Check sheet for the modelled part. Datum: model origin and axes. Units: mm. Coordinates: 2 decimals unless noted, no trailing zeros. Loops run counter-clockwise (first coordinate to the right, second up) from the corner with the lowest first, then second, coordinate; pieces in that order, holes last. Notation, with made-up numbers: M 44,71.5 L 85,71.5 A16 ccw 85,93.5 Z; hole C -32.5,67 d9. An arc over 180 degrees is marked long. Answer in a Markdown table with one row per item. Add a question column.
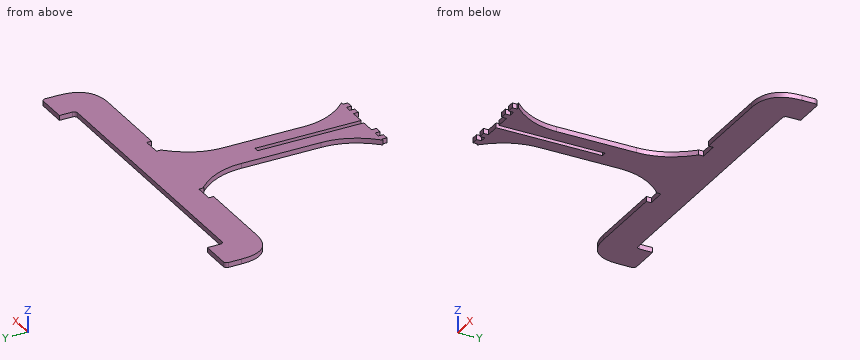
```python
from build123d import *

# Parameters (mm, degrees)
P_IDAT_VYSUNUT_M2_DEPTH  = 3
SKICA2_W                 = 3
SKICA2_H                 = 65
ODEBRAT_VYSUNUT_M3_DEPTH = 3
SKICA3_W                 = 11
SKICA3_H                 = 5.694256757
ODEBRAT_VYSUNUT_M4_DEPTH = 3


with BuildPart() as part:
    # Skica1 → Přidat vysunutím2 (new body)
    with BuildSketch(Plane.XY):
        with BuildLine():
            Line((-90.642636358, 2.694256757), (-30.642636358, 2.694256757))
            add(Edge.make_bspline(
                [(-30.642636358, 2.694256757), (-17.025139471, -11.118063286), (-17.142636358, -27.878389443)],
                knots=[0, 0, 0, 1, 1, 1], degree=2))
            Line((-17.142636358, -27.878389443), (-17.142636358, -76.655981804))
            add(Edge.make_bspline(
                [(-30.642636358, -107.305743243), (-17.009316786, -93.458261678), (-17.142636358, -76.655981804)],
                knots=[0, 0, 0, 1, 1, 1], degree=2))
            Line((-30.642636358, -107.305743243), (-29.497972973, -107.305743243))
            Line((-29.497972973, -107.305743243), (-29.497972973, -110.305743243))
            Line((-29.497972973, -110.305743243), (-25.347972973, -110.305743243))
            Line((-25.347972973, -110.305743243), (-25.347972973, -107.305743243))
            Line((-25.347972973, -107.305743243), (-21.697972973, -107.305743243))
            Line((-21.697972973, -107.305743243), (-21.697972973, -110.305743243))
            Line((-21.697972973, -110.305743243), (-17.547972973, -110.305743243))
            Line((-17.547972973, -110.305743243), (-17.547972973, -107.305743243))
            Line((-17.547972973, -107.305743243), (2.852027027, -107.305743243))
            Line((2.852027027, -107.305743243), (2.852027027, -110.305743243))
            Line((2.852027027, -110.305743243), (7.002027027, -110.305743243))
            Line((7.002027027, -110.305743243), (7.002027027, -107.305743243))
            Line((7.002027027, -107.305743243), (10.652027027, -107.305743243))
            Line((10.652027027, -107.305743243), (10.652027027, -110.305743243))
            Line((10.652027027, -110.305743243), (14.802027027, -110.305743243))
            Line((14.802027027, -110.305743243), (14.802027027, -107.305743243))
            Line((14.802027027, -107.305743243), (16.357363642, -107.305743243))
            add(Edge.make_bspline(
                [(16.357363642, -107.305743243), (2.72404407, -93.458261678), (2.857363642, -76.655981804)],
                knots=[0, 0, 0, 1, 1, 1], degree=2))
            Line((2.857363642, -76.655981804), (2.857363642, -27.878389443))
            add(Edge.make_bspline(
                [(16.357363642, 2.694256757), (2.739866756, -11.118063286), (2.857363642, -27.878389443)],
                knots=[0, 0, 0, 1, 1, 1], degree=2))
            Line((16.357363642, 2.694256757), (76.357363642, 2.694256757))
            add(Edge.make_bspline(
                [(96.357363642, 22.694256757), (96.357363642, 2.694256757), (76.357363642, 2.694256757)],
                knots=[0, 0, 0, 1, 1, 1], degree=2))
            Line((96.357363642, 22.694256757), (96.357363642, 30.694256757))
            ThreePointArc((96.357363642, 30.694256757), (95.771577204, 32.108470319), (94.357363642, 32.694256757))
            Line((94.357363642, 32.694256757), (76.357363642, 32.694256757))
            Line((76.357363642, 32.694256757), (76.357363642, 24.694256757))
            ThreePointArc((76.357363642, 24.694256757), (75.771577204, 23.280043194), (74.357363642, 22.694256757))
            Line((74.357363642, 22.694256757), (-88.642636358, 22.694256757))
            ThreePointArc((-88.642636358, 22.694256757), (-90.05684992, 23.280043194), (-90.642636358, 24.694256757))
            Line((-90.642636358, 24.694256757), (-90.642636358, 32.694256757))
            Line((-90.642636358, 32.694256757), (-108.642636358, 32.694256757))
            ThreePointArc((-108.642636358, 32.694256757), (-110.05684992, 32.108470319), (-110.642636358, 30.694256757))
            Line((-110.642636358, 30.694256757), (-110.642636358, 22.694256757))
            add(Edge.make_bspline(
                [(-110.642636358, 22.694256757), (-110.642636358, 2.694256757), (-90.642636358, 2.694256757)],
                knots=[0, 0, 0, 1, 1, 1], degree=2))
        make_face()
    extrude(amount=P_IDAT_VYSUNUT_M2_DEPTH)

    # Skica2 → Odebrat vysunutím3 (cut)
    with BuildSketch(Plane(origin=(0, 0, 0), x_dir=(-1, 0, 0), z_dir=(0, 0, -1))):
        with Locations((7.347972973, -74.805743243)):
            Rectangle(SKICA2_W, SKICA2_H)
    extrude(amount=-ODEBRAT_VYSUNUT_M3_DEPTH, mode=Mode.SUBTRACT)

    # Skica3 → Odebrat vysunutím4 (cut)
    with BuildSketch(Plane(origin=(0, 0, 0), x_dir=(-1, 0, 0), z_dir=(0, 0, -1))):
        with Locations((-22.152027027, 2.847128379)):
            Rectangle(SKICA3_W, SKICA3_H)
        with Locations((36.847972973, 2.847128379)):
            Rectangle(SKICA3_W, SKICA3_H)
    extrude(amount=-ODEBRAT_VYSUNUT_M4_DEPTH, mode=Mode.SUBTRACT)


solid = part.part
```
Q1. Thickness scan on L1, parallel to X at y = -50, z = 1.8; L2, parallel to Y at x = -33.5, z = 2.15; L3, parallel to Y at x = -49.5, z = 2.85. Record the ranges inside material, lowest first.
Q2. Go/stop test with flat-tipped pins: pin 1 (0.9 mm diameter, centred on y = -109.5, z = 1, fed in from +X); pin 2 (1.5 mm diameter, centred on x = 59, z = 1.5, fed in from -Y); pin 3 (0.9 mm diameter, centred on y = -71.5, z = 1.5, fed in from -X). Record where each tip stops, or that it passes through.
Q3. Cross-section at A-A (y = -62.5). Record the cut outline in (x, z).
Q4. Cross-section at B-B (x = -47.5). Record the cut outline in (y, z).
Answer key:
| question | item | result |
|---|---|---|
| 1 | L1 | -17.14 to -8.85, -5.85 to 2.86 |
| 1 | L2 | 5.69 to 22.69 |
| 1 | L3 | 2.69 to 22.69 |
| 2 | pin 1 | x = 14.8 |
| 2 | pin 2 | y = 2.69 |
| 2 | pin 3 | x = -17.14 |
| 3 | outline | M -17.14,0 L -8.85,0 L -8.85,3 L -17.14,3 Z; M -5.85,0 L 2.86,0 L 2.86,3 L -5.85,3 Z |
| 4 | outline | M 2.69,0 L 22.69,0 L 22.69,3 L 2.69,3 Z |
